```python
from build123d import *

# Parameters (mm, degrees)
EXTRUDE_1_DEPTH     = 2
SKETCH_2_R          = 2
CUT_EXTRUDE_1_DEPTH = 2
FILLET_1_R          = 2


with BuildPart() as part:
    # 草图1 → 凸台-拉伸1 (new body)
    with BuildSketch(Plane.XY):
        with BuildLine():
            Line((0, 0), (0, -45))
            Line((0, -45), (-20, -45))
            Line((-20, -45), (-20, -35))
            ThreePointArc((-20, -35), (-24.393398282, -24.393398282), (-35, -20))
            Line((-35, -20), (-45, -20))
            Line((-45, -20), (-45, 0))
            Line((-45, 0), (0, 0))
        make_face()
    extrude(amount=EXTRUDE_1_DEPTH)

    # 草图2 → 切除-拉伸1 (cut)
    with BuildSketch(Plane.XY.offset(2)):
        with Locations((-10, -40)):
            Circle(SKETCH_2_R)
        with Locations((-10, -25)):
            Circle(SKETCH_2_R)
        with Locations((-25, -10)):
            Circle(SKETCH_2_R)
        with Locations((-40, -10)):
            Circle(SKETCH_2_R)
    extrude(amount=-CUT_EXTRUDE_1_DEPTH, mode=Mode.SUBTRACT)

    # 圆角1
    fillet_1_edges = [part.edges().sort_by_distance(p)[0] for p in [
        (0, 0, 1),
        (0, -45, 1),
        (-20, -45, 1),
        (-45, -20, 1),
        (-45, 0, 1),
    ]]
    fillet(fillet_1_edges, radius=FILLET_1_R)


solid = part.part
```
Build history of the part. All positions in model axes, mm. A direction names the side the tool comes from. Coordinates: 2 decimals unless noted, no trailing zeros. Order: outer loops, then holes, each group sorted by start corner. A loop starts at its lowest first (then second) coordinate and runs counter-clockwise, first axis right, second up.
Item 1: Mould opens along Y. For faces 3 (the flat face through (-20, -39, 1)), 4 (the cylindrical face through (-42, -10, 1)), 5 (the flat face through (-23, 0, 1)) say: released by +Y, released by -Y, zero draft, split by the parting line, or undercut.
Filled in:
face 3: zero draft
face 4: undercut
face 5: released by +Y
Item 2: Drop flat-ended pins along their axis: pin 1 Ø3.5 at (x, y) = (-10, -40) entering from +Z; pin 2 Ø1 at (y, z) = (-40, 0.5) entering from -X. Give the stop position or say it passes through.
Filled in:
pin 1: passes through
pin 2: stops at x = -20
Item 3: Drill centre lines: L1, parallel to Y at x = -10, z = 0.9; L2, parallel to X at y = -9, z = 0.1; L3, parallel to X at y = -35, z = 1.7. Where is each one in solid material? Low to high.
Filled in:
L1: y = -45 to -42, -38 to -27, -23 to 0
L2: x = -45 to -41.73, -38.27 to -26.73, -23.27 to 0
L3: x = -20 to 0
Item 4: Saw through at A-A on x = -10. List the corners of the cut face in (y, z).
Filled in:
outline: (-45, 0) - (-42, 0) - (-42, 2) - (-45, 2) - close; (-38, 0) - (-27, 0) - (-27, 2) - (-38, 2) - close; (-23, 0) - (0, 0) - (0, 2) - (-23, 2) - close
Item 5: Saw through at D-D on z = 1.35. List the corners of the cut face in (x, y).
Filled in:
outline: (-45, -18) arc R2 ccw to (-43, -20) - (-35, -20) arc R15 cw to (-20, -35) - (-20, -43) arc R2 ccw to (-18, -45) - (-2, -45) arc R2 ccw to (0, -43) - (0, -2) arc R2 ccw to (-2, 0) - (-43, 0) arc R2 ccw to (-45, -2) - close; hole circle Ø4 at (-40, -10); hole circle Ø4 at (-25, -10); hole circle Ø4 at (-10, -40); hole circle Ø4 at (-10, -25)
Item 6: Tool access for faces 1 (the cylindrical face through (-11.6, -26.2, 1)), 2 (the flat face through (-39, -20, 1)): list every direction of +Z, -Z, +X, -X, +Y, -Y with a clear straight run to the whole face (end or side of a thin tool).
Filled in:
face 1: +Z, -Z
face 2: +Z, -Z, -X, -Y
Item 7: Saw through at C-C on y = -40. List the corners of the cut face in (x, z), then the cut area to 3 significant figures.
Filled in:
outline: (-20, 0) - (-12, 0) - (-12, 2) - (-20, 2) - close; (-8, 0) - (0, 0) - (0, 2) - (-8, 2) - close
area: 32.0 mm2
